For this review, take the finished solid that the model builds, in its own axes (mm). A direction names the side the tool comes from. Round coordinates to 2 decimals unless told otherwise and drop trailing zeros. Loops run counter-clockwise (first coordinate to the right, second up) from the corner with the lowest first, then second, coordinate; pieces in that order, holes last.
1. Draft analysis for pull direction Y (two halves, no side actions). For faces 1 (the flat face through (-212.53, 114.96, 8.87)), 2 (the cylindrical face through (5.9, 21, 8.9)), 3 (the flat face through (-1, 236, 0)), state which applies: released by +Y, released by -Y, zero draft, split by the parting line, or undercut.
2. Consider section C-C on x = 202.5. State the section outline as (y, z) points, then the cut area to 3 significant figures.
3. Tool access review of faces 4 (the flat face through (77.878, 53.664, 9.126)), 5 (the flat face through (213.175, 116.59, 8.874)): name each direction out of +Z, -Z, +X, -X, +Y, -Y from which nothing blocks a thin tool from reaching the whole face with its end or side.
4. To check wall thickness, follow line 1 along Y through (x, z) = (-96.5, 6.25); line 2 along Y through (x, z) = (81.5, 6.75); line 3 along X through (y, z) = (178, 3.75). State the ranges of each line that lie inside material, in increasing order.
5. Consider section A-A on x = 25. State the section outline as (y, z) points.
6. Consider section B-B on y = 151.5. State the section outline as (x, z) points, then the cut area to 3 significant figures.
7. Clearance check with flat-ended pins moving along their axes: pin 1 Ø6 at (x, z) = (118, 9.5) entering from +Y; pin 2 Ø1 at (x, z) = (-96, 15) entering from +Y; pin 3 Ø3 at (x, z) = (-94, 13) entering from +Y; pin 4 Ø2 at (x, y) = (163, 216) entering from -Z. State where each tip first meets the part, or that it passes through.
Autodesk Inventor part; units mm, degrees
ref_plane "YZ Plane" through (0, 0, 0) normal (1, 0, 0) x (0, 1, 0)
ref_plane "XZ Plane" through (0, 0, 0) normal (0, 1, 0) x (-1, 0, 0)
ref_plane "XY Plane" through (0, 0, 0) normal (0, 0, 1) x (1, 0, 0)
sketch "Sketch1" plane through (0, 0, 0) normal (0, 0, 1) x (1, 0, 0)
  line L0 (0, 9.7536) -> (-185.3184, 46.3296)
  line L1 (-185.3184, 46.3296) -> (-240.1824, 184.7088)
  line L2 (-240.1824, 184.7088) -> (0, 272.1864)
  line L3 (0, 562.8605) -> (0, -145.2705) construction
  line L4 (0, 272.1864) -> (0, 9.7536)
  point P0 (0, 0)
  dimension "d9" = 272.1864
  dimension "d11" = 240.1824
  dimension "d15" = 184.7088
  dimension "d20" = 185.3184
  dimension "d22" = 46.3296
  dimension "d39" = 0
  dimension "d41" = 0
  dimension "d42" = 9.7536
extrude "Extrusion4" add sketch "Sketch1" along normal blind 18
hole "Hole2" at (0.0182, 265.1521, 18) direction (0, 0, -1) diameter 15 end through all
hole "Hole3" at (-233.7862, 182.8308, 18) direction (0, 0, -1) diameter 15 end through all
hole "Hole4" at (-180.9047, 51.7876, 18) direction (0, 0, -1) diameter 15 end through all
hole "Hole5" at (0.2097, 16.6506, 18) direction (0, 0, -1) diameter 15 end through all
sketch "Sketch6" plane through (0, 0, 18) normal (0, 0, 1) x (1, 0, 0)
  line L0 (-30, 231.4607) -> (-208.2387, 166.5438)
  line L1 (-208.2387, 166.5438) -> (-170.7523, 71.9949)
  line L2 (-170.7523, 71.9949) -> (-30, 44.2148)
  line L3 (-5.5654, 270.1594) -> (-229.1506, 188.7267)
  line L4 (-236.6974, 175.9189) -> (-188.1895, 53.5712)
  line L5 (-177.9802, 44.8813) -> (-4.1975, 10.582)
  line L6 (0, 231.4607) -> (-30, 231.4607)
  line L7 (0, 44.2148) -> (-30, 44.2148)
  line L8 (0, 44.2148) -> (0, 231.4607)
  point P0 (0, 0)
  dimension "d167" = 23
  dimension "d168" = 28
  dimension "d170" = 28
  dimension "d171" = 30
  dimension "d173" = 0
  dimension "d174" = 30
extrude "Extrusion6" cut sketch "Sketch6" against normal through all
fillet "Fillet6" radius 40 1 edges at (-208.2387, 166.5438, 9)
fillet "Fillet7" radius 100 1 edges at (-170.7523, 71.9949, 9)
fillet "Fillet8" radius 100 1 edges at (-30, 44.2148, 9)
fillet "Fillet9" radius 100 1 edges at (-30, 231.4607, 9)
fillet "Fillet10" radius 1.5 1 edges at (-5.5654, 270.1594, 9)
fillet "Fillet11" radius 1 1 edges at (-229.1506, 188.7267, 9)
fillet "Fillet12" radius 1 1 edges at (-236.6974, 175.9189, 9)
fillet "Fillet13" radius 2 1 edges at (-177.9802, 44.8813, 9)
fillet "Fillet14" radius 2 1 edges at (-188.1895, 53.5712, 9)
fillet "Fillet15" radius 2 1 edges at (-4.1975, 10.582, 9)
mirror "Mirror3" about plane through (0, 0, 0) normal (1, 0, 0)
properties part number "section1" material "Polyethylene, High Density"
Resolved:
1. face 1: released by -Y
1. face 2: undercut
1. face 3: zero draft
2. outline: (89.67, 0) - (198.43, 0) - (198.43, 18) - (89.67, 18) - close
2. area: 1,960 mm2
3. face 4: +Z, -Z
3. face 5: +Z, -Z, +X, -Y
4. line 1: y = 28.8 to 57.34, 207.24 to 237.04
4. line 2: y = 25.84 to 54.38, 212.7 to 242.5
4. line 3: x = -228.05 to -175.33, 175.33 to 228.05
5. outline: (14.69, 0) - (44.33, 0) - (44.33, 18) - (14.69, 18) - close; (230.66, 0) - (263.08, 0) - (263.08, 18) - (230.66, 18) - close
6. outline: (-227.02, 0) - (-194.99, 0) - (-194.99, 18) - (-227.02, 18) - close; (194.99, 0) - (227.02, 0) - (227.02, 18) - (194.99, 18) - close
6. area: 1,150 mm2
7. pin 1: stops at y = 230.3
7. pin 2: stops at y = 237.4
7. pin 3: stops at y = 238.5
7. pin 4: passes through
